Design review of the part built by this model. Coordinates are the model's own, in mm. A direction names the side the tool comes from. Give positions to 0.01 mm unless a question says otherwise; leave off trailing zeros. Order: outer loops, then holes, each group sorted by start corner. A loop starts at its lowest first (then second) coordinate and runs counter-clockwise, first axis right, second up. Notation, with made-up numbers: M 9,6 L 63,6 A31 cw 63,39 Z; hole C 26.5,22.5 d1. An arc over 180 degrees is marked long. Answer as a JSON object with one key per item and string values.
Autodesk Inventor part; units mm, degrees
ref_plane "YZ Plane" through (0, 0, 0) normal (1, 0, 0) x (0, 1, 0)
ref_plane "XZ Plane" through (0, 0, 0) normal (0, 1, 0) x (-1, 0, 0)
sketch "Sketch1" plane through (0, 0, 0) normal (0, 1, 0) x (-1, 0, 0)
  circle A0 centre (0, 0) radius 3.575
  circle A1 centre (0, 0) radius 5
  dimension "d0" = 7.15
  dimension "d1" = 10
extrude "Extrusion1" add sketch "Sketch1" along normal mid plane 40
ref_plane "Work Plane1" through (0, 0, 5) normal (0, 0, 1) x (1, 0, 0)
sketch "Sketch2" plane through (0, 0, 5) normal (0, 0, 1) x (1, 0, 0)
  circle A0 centre (0, 0) radius 3.575
  circle A1 centre (0, 0) radius 5
  line L0 (5, 20) -> (-5, 20)
  dimension "d4" = 7.15
  dimension "d5" = 10
  dimension "d22" = 0
extrude "Extrusion2" add sketch "Sketch2" along normal blind 15 and the other way blind 5
sketch "Sketch3" plane through (0, 0, 20) normal (0, 0, 1) x (1, 0, 0)
  circle A0 centre (0, 0) radius 3.575
extrude "Extrusion3" cut sketch "Sketch3" against normal up to surface
sketch "Sketch4" plane through (0, 20, 0) normal (0, 1, 0) x (1, 0, 0)
  circle A0 centre (0, 0) radius 3.615
  dimension "d13" = 7.23
extrude "Extrusion4" cut sketch "Sketch4" against normal through all
sketch "Sketch5" plane through (0, 0, -5) normal (0, 0, 1) x (1, 0, 0)
  line L0 (5, 15) -> (-5, 15)
  line L1 (-5, -15) -> (5, -15)
  line L2 (2, 15) -> (-2, 15)
  line L3 (-2, 15) -> (-2, -15)
  line L4 (-2, -15) -> (2, -15)
  line L5 (2, -15) -> (2, 15)
  point P0 (0, 0)
  dimension "d16" = 4
  dimension "d17" = 2
properties part number "T-joint"
(1) Tool access review of faces 4 (the cylindrical face through (-4, 3, 12)), 5 (the flat face through (-3, 20, 3)): name each direction out of +Z, -Z, +X, -X, +Y, -Y from which nothing blocks a thin tool from reaching the whole face with its end or side.
Checked values:
{"face 4": "+Z", "face 5": "+Z, -Z, +X, -X, +Y"}
(2) We need section A-A (x = 0). Write out the cut boundary in (y, z) (3 decimals), plus the area to 3 significant figures.
Checked values:
{"outline": "M -20,-5 L 20,-5 L 20,-3.615 L -20,-3.615 Z; M -20,3.615 L -3.575,3.615 L -3.575,20 L -5,20 L -5,5 L -20,5 Z; M 3.575,3.615 L 20,3.615 L 20,5 L 5,5 L 5,20 L 3.575,20 Z", "area": "144 mm^2"}
(3) Insertion check: pin 1 (3 mm diameter, centred on x = 3, z = 15, fed in from +Y); pin 2 (1.5 mm diameter, centred on x = -3, z = 14, fed in from +Y); pin 3 (6 mm diameter, centred on x = 1, z = 13, fed in from +Y). Each pin has a flat end and moves straight along its axis. Give the tip position at first contact, or say it passes through.
Checked values:
{"pin 1": "stops at y = 4.77", "pin 2": "stops at y = 4.47", "pin 3": "stops at y = 5"}
(4) We need section B-B (z = 2.75). Write out the cut boundary in (x, y) (3 decimals).
Checked values:
{"outline": "M -4.176,-20 L -2.346,-20 L -2.346,-2.697 A3.575 cw -2.346,2.697 L -2.346,20 L -4.176,20 L -4.176,2.75 A5 ccw -4.176,-2.75 Z; M 2.346,-20 L 4.176,-20 L 4.176,-2.75 A5 ccw 4.176,2.75 L 4.176,20 L 2.346,20 L 2.346,2.697 A3.575 cw 2.346,-2.697 Z"}
(5) To check wall thickness, follow L1, parallel to Y at x = 0, z = 16.75 (3 decimals); L2, parallel to X at y = -6, z = 0 (3 decimals). State the ranges of each line that lie inside material, in increasing order. Write a range as from..to.
Checked values:
{"L1": "y = -5..-3.575, 3.575..5", "L2": "x = -5..-3.615, 3.615..5"}
(6) Draft analysis for pull direction Z (two halves, no side actions). For faces 1 (the cylindrical face through (0.651, -0.28, -4.957)), 2 (the cylindrical face through (-0.471, 0.28, -3.584)), 3 (the flat face through (3.3, -2.2, 20)), state which applies: +Z half, -Z half, draft (parallel to the pull), parting line (faces both ways), or undercut.
Checked values:
{"face 1": "parting line", "face 2": "undercut", "face 3": "+Z half"}
(7) We need section D-D (z = 13). Write out the cut boundary in (x, y) (3 decimals), plus the area to 3 significant figures.
Checked values:
{"outline": "C 0,0 d10; hole C 0,0 d7.15", "area": "38.4 mm^2"}
